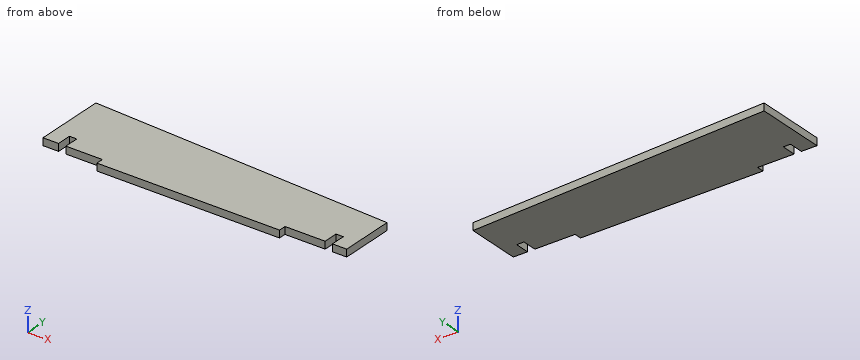
Autodesk Inventor part; units mm, degrees
ref_plane "YZ Plane" through (0, 0, 0) normal (1, 0, 0) x (0, 1, 0)
ref_plane "XZ Plane" through (0, 0, 0) normal (0, 1, 0) x (-1, 0, 0)
ref_plane "XY Plane" through (0, 0, 0) normal (0, 0, 1) x (1, 0, 0)
sketch "Sketch1" plane through (0, 0, 0) normal (0, 0, 1) x (1, 0, 0)
  line L0 (-64, 50) -> (64, 50)
  line L1 (64, 50) -> (64, 0)
  line L2 (64, 0) -> (-64, 0)
  line L3 (-64, 0) -> (-64, 50)
  line L4 (-25, 0) -> (25, 0)
  line L5 (25, 0) -> (25, -2)
  line L6 (25, -2) -> (-25, -2)
  line L7 (-25, -2) -> (-25, 0)
  point P0 (0, 0)
  point P1 (0, 0)
  dimension "d0" = 50
  dimension "d1" = 128
  dimension "d2" = 2
  dimension "d3" = 50
extrude "Extrusion1" add sketch "Sketch1" along normal mid plane 2
sketch "Sketch2" plane through (0, 0, 1) normal (0, 0, 1) x (1, 0, 0)
  line L0 (-37.004, 19.1647) -> (37.8795, 15.001)
  line L1 (37.8795, 15.001) -> (37.8795, 6.0072)
  line L2 (37.8795, 6.0072) -> (-37.004, 10.1709)
  line L3 (-37.004, 10.1709) -> (-37.004, 19.1647)
  line L4 (-41.259, 17.7892) -> (-41.259, 8.0268)
  line L5 (41.9117, 3.4023) -> (41.9117, 13.1647)
  point P0 (0, 0)
sketch "Sketch3" plane through (0, 0, 1) normal (0, 0, 1) x (1, 0, 0)
  line L0 (-41.259, 17.7892) -> (-41.259, 8.0268) construction
  line L1 (-37.004, 19.1647) -> (37.8795, 15.001) construction
  line L2 (41.9117, 3.4023) -> (41.9117, 13.1647) construction
  line L3 (-41.259, 19.4013) -> (41.9117, 14.7768)
  line L4 (41.9117, 14.7768) -> (41.9117, 0)
  line L5 (91.9117, 0) -> (91.9117, 60)
  line L6 (91.9117, 60) -> (-91.259, 60)
  line L7 (-91.259, 60) -> (-91.259, 0)
  line L8 (-91.259, 0) -> (-41.259, 0)
  line L9 (-41.259, 0) -> (-41.259, 19.4013)
  line L10 (41.9117, 0) -> (91.9117, 0)
  point P0 (0, 0)
  dimension "d6" = 60
  dimension "d7" = 50
  dimension "d8" = 50
extrude "Extrusion2" cut sketch "Sketch3" against normal through all
sketch "Sketch4" plane through (0, 0, 1) normal (0, 0, 1) x (1, 0, 0)
  line L0 (36, 15.6306) -> (36, 0)
  line L1 (38, 15.6306) -> (36, 15.6306)
  line L2 (38, 0) -> (38, 15.6306)
  line L3 (36, 0) -> (38, 0)
  line L4 (-37, 19.7943) -> (-37, 0)
  line L5 (-35, 19.7943) -> (-37, 19.7943)
  line L6 (-35, 0) -> (-35, 19.7943)
  line L7 (-37, 0) -> (-35, 0)
  point P0 (0, 0)
sketch "Sketch5" plane through (0, 0, 1) normal (0, 0, 1) x (1, 0, 0)
  line L0 (-37, 19.7943) -> (-37, 0) construction
  line L1 (-35, 0) -> (-35, 19.7943) construction
  line L2 (36, 15.6306) -> (36, 0) construction
  line L3 (38, 0) -> (38, 15.6306) construction
  line L4 (-37, 4) -> (-35, 4)
  line L5 (-35, 4) -> (-35, 0)
  line L6 (-35, 0) -> (-37, 0)
  line L7 (-37, 0) -> (-37, 4)
  line L8 (38, 4) -> (36, 4)
  line L9 (36, 4) -> (36, 0)
  line L10 (36, 0) -> (38, 0)
  line L11 (38, 0) -> (38, 4)
  point P0 (0, 0)
  dimension "d11" = 4
  dimension "d12" = 4
extrude "Extrusion3" cut sketch "Sketch5" against normal through all
properties part number "angle_plate_short_tall"
Model file for the job. Use its own axes, mm. Coordinates: 2 decimals unless noted, no trailing zeros. Order: outer loops, then holes, each group sorted by start corner. A loop starts at its lowest first (then second) coordinate and runs counter-clockwise, first axis right, second up. Notation, with made-up numbers: (20, -11) -> (35, -11) arc R20 ccw to (35, 24) -> close; hole circle Ø11 at (57.25, 74). An arc over 180 degrees is marked (long way). Return JSON: item names as keys, results as strings.
Item 1: Slice it at A-A (y = 0.75). Write the cut outline in (x, z).
Model answer:
{"outline": "(-41.26, -1) -> (-37, -1) -> (-37, 1) -> (-41.26, 1) -> close; (-35, -1) -> (36, -1) -> (36, 1) -> (-35, 1) -> close; (38, -1) -> (41.91, -1) -> (41.91, 1) -> (38, 1) -> close"}
Item 2: Slice it at B-B (z = 0.65). Write the cut outline in (x, y).
Model answer:
{"outline": "(-41.26, 0) -> (-37, 0) -> (-37, 4) -> (-35, 4) -> (-35, 0) -> (-25, 0) -> (-25, -2) -> (25, -2) -> (25, 0) -> (36, 0) -> (36, 4) -> (38, 4) -> (38, 0) -> (41.91, 0) -> (41.91, 14.78) -> (-41.26, 19.4) -> close"}
Item 3: Slice it at D-D (y = 15.5). Write the cut outline in (x, z).
Model answer:
{"outline": "(-41.26, -1) -> (28.91, -1) -> (28.91, 1) -> (-41.26, 1) -> close"}
Item 4: Slice it at C-C (x = -11.5). Write the cut outline in (y, z).
Model answer:
{"outline": "(-2, -1) -> (17.75, -1) -> (17.75, 1) -> (-2, 1) -> close"}
Item 5: Pin check, flat tips, straight feed: P1, Ø1, axis at x = 39.5, z = 0, coming from the -Y side; P2, Ø1, axis at x = -12.5, z = -0.5, coming from the +Y side; P3, Ø0.6, axis at x = 36.5, z = 0, coming from the -Y side. Stop position of each tip, or through.
Model answer:
{"P1": "stops at y = 0", "P2": "stops at y = 17.83", "P3": "stops at y = 4"}
Item 6: Wall check: line 1 along X through (y, z) = (1, -0.25); line 2 along Y through (x, z) = (24.5, 0.95); line 3 along Y through (x, z) = (-32.5, 0.95). Give the ranges that are in metal, low to high. Write a range as from..to.
Model answer:
{"line 1": "x = -41.26..-37, -35..36, 38..41.91", "line 2": "y = -2..15.74", "line 3": "y = 0..18.91"}
